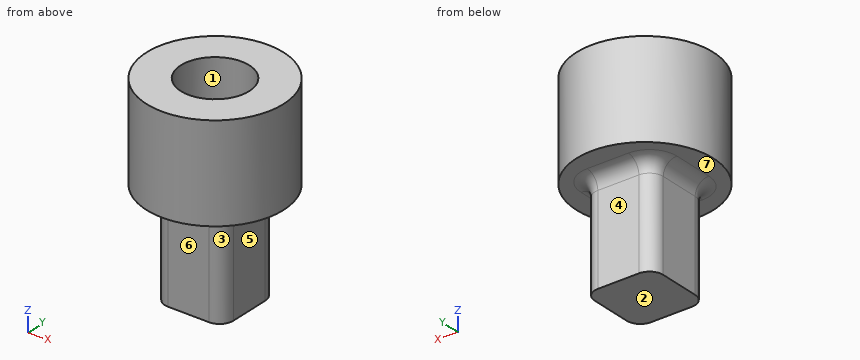
```python
from build123d import *

# Parameters (mm, degrees)
BOSS_EXTRUDE1_DEPTH = 7.5
SKETCH2_R           = 5
BOSS_EXTRUDE2_DEPTH = 2
SKETCH3_R           = 5
SKETCH3_R_2         = 2.5
BOSS_EXTRUDE3_DEPTH = 5
FILLET1_R           = 1


with BuildPart() as part:
    # Sketch1 → Boss-Extrude1 (new body)
    with BuildSketch(Plane.XY):
        with BuildLine():
            Line((-1.5, -2.5), (1.5, -2.5))
            ThreePointArc((1.5, -2.5), (2.207106781, -2.207106781), (2.5, -1.5))
            Line((2.5, -1.5), (2.5, 1.5))
            ThreePointArc((2.5, 1.5), (2.207106781, 2.207106781), (1.5, 2.5))
            Line((1.5, 2.5), (-1.5, 2.5))
            ThreePointArc((-1.5, 2.5), (-2.207106781, 2.207106781), (-2.5, 1.5))
            Line((-2.5, 1.5), (-2.5, -1.5))
            ThreePointArc((-2.5, -1.5), (-2.207106781, -2.207106781), (-1.5, -2.5))
        make_face()
    extrude(amount=BOSS_EXTRUDE1_DEPTH)

    # Sketch2 → Boss-Extrude2 (add)
    with BuildSketch(Plane.XY.offset(7.5)):
        Circle(SKETCH2_R)
    extrude(amount=BOSS_EXTRUDE2_DEPTH)

    # Sketch3 → Boss-Extrude3 (add)
    with BuildSketch(Plane.XY.offset(9.5)):
        Circle(SKETCH3_R)
        Circle(SKETCH3_R_2, mode=Mode.SUBTRACT)
    extrude(amount=BOSS_EXTRUDE3_DEPTH)

    # Fillet1
    fillet1_edges = [part.edges().sort_by_distance(p)[0] for p in [
        (-2.207106781, 2.207106781, 7.5),
        (-2.5, 0, 7.5),
        (-2.207106781, -2.207106781, 7.5),
        (0, -2.5, 7.5),
        (2.207106781, -2.207106781, 7.5),
        (2.5, 0, 7.5),
        (2.207106781, 2.207106781, 7.5),
        (0, 2.5, 7.5),
    ]]
    fillet(fillet1_edges, radius=FILLET1_R)


solid = part.part
```
Source: CAD feature listing. Evaluate the final solid. Frame: model axes, mm. Face numbers are marked on the shaded views. A direction names the side the tool comes from. Give positions to 0.01 mm unless a question says otherwise; leave off trailing zeros. Order: outer loops, then holes, each group sorted by start corner. A loop starts at its lowest first (then second) coordinate and runs counter-clockwise, first axis right, second up. Notation, with made-up numbers: (83, 28) -> (122, 28) arc R15 ccw to (122, 42) -> close; hole circle Ø4 at (71, 87.5). An arc over 180 degrees is marked (long way). Use a Markdown table: item, result.
Q1. First-contact query: P1, Ø3.5, axis at x = 0, z = 2.5, coming from the +Y side; P2, Ø1.5, axis at x = -2, z = 7.5, coming from the -Y side; P3, Ø0.9, axis at y = 0.5, z = 2.5, coming from the +X side. Flat tips, straight axial feed; report the tip coordinate or a pass-through.
A:
| item | result |
|---|---|
| P1 | y = 2.5 |
| P2 | y = -4.84 |
| P3 | x = 2.5 |
Q2. Access query for the marked faces 4, 5, 6 and 7. Directions: +Z, -Z, +X, -X, +Y, -Y. A direction counts if a zero-diameter tool reaches every point of the face in a straight line with its end or side. Return the directions, or none.
A:
| item | result |
|---|---|
| face 4 | -Z, +X, -X, +Y |
| face 5 | -Z, +X, +Y, -Y |
| face 6 | -Z, +X, -X, -Y |
| face 7 | -Z |
Q3. Pull-direction query (X, two-part tool) for the marked faces 1, 2 and 3; classes: +X half, -X half, draft (parallel to the pull), parting line (faces both ways), or undercut.
A:
| item | result |
|---|---|
| face 1 | undercut |
| face 2 | draft |
| face 3 | +X half |
Q4. Section A-A (y = 0). Return the cut outline in (x, z).
A:
| item | result |
|---|---|
| outline | (-5, 7.5) -> (-3.5, 7.5) arc R1 cw to (-2.5, 6.5) -> (-2.5, 0) -> (2.5, 0) -> (2.5, 6.5) arc R1 cw to (3.5, 7.5) -> (5, 7.5) -> (5, 14.5) -> (2.5, 14.5) -> (2.5, 9.5) -> (-2.5, 9.5) -> (-2.5, 14.5) -> (-5, 14.5) -> close |
Q5. Material intervals for line 1 (Y direction, x = 0, z = 11.3); line 2 (Z direction, x = -1.25, y = -3.75); line 3 (Y direction, x = 1.5, z = 2.75), sorted ascending. Write a range as [from, to].
A:
| item | result |
|---|---|
| line 1 | [-5, -2.5], [2.5, 5] |
| line 2 | [7.5, 14.5] |
| line 3 | [-2.5, 2.5] |
Q6. Section C-C (z = 9.25). Return the cut outline in (x, y), and give its area (3 significant figures).
A:
| item | result |
|---|---|
| outline | circle Ø10 at (0, 0) |
| area | 78.5 mm^2 |
